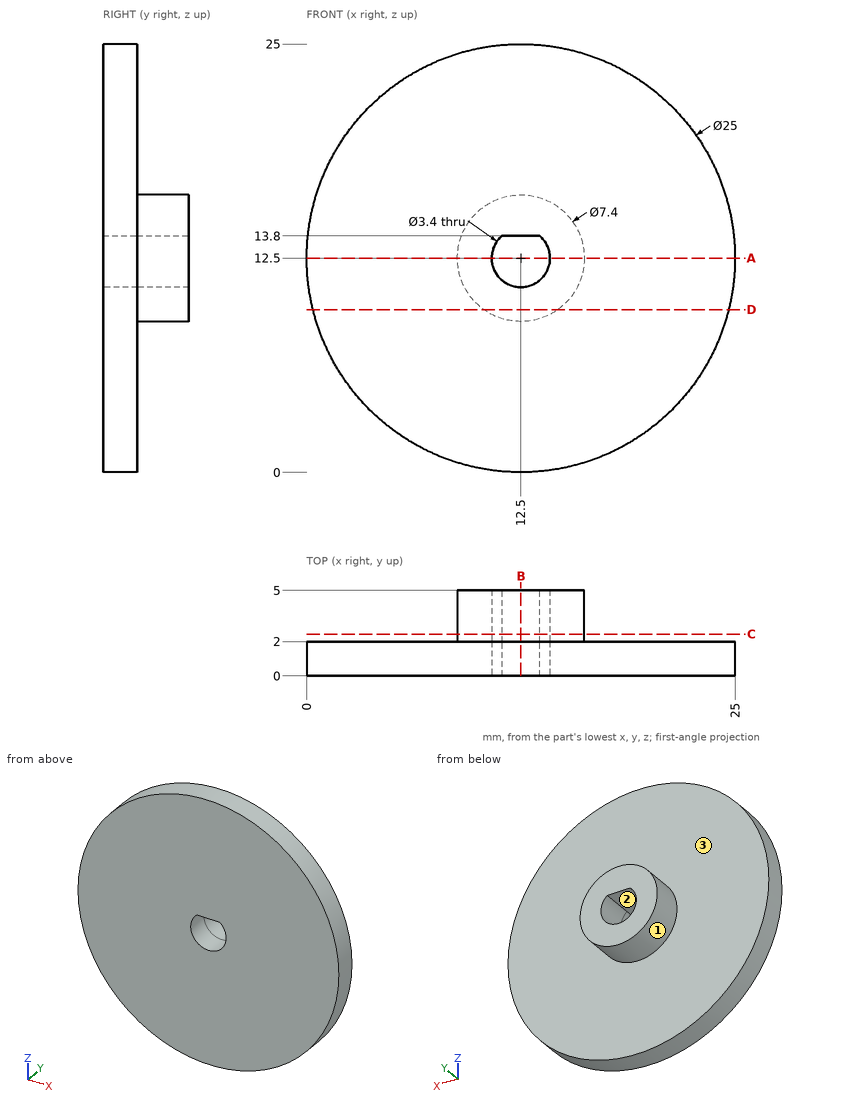
Design review of the part shown in the three views and the two pictorial views. Dimensions are in mm from the part's minimum x, y and z. Round coordinates to 2 decimals unless told otherwise and drop trailing zeros. Loops run counter-clockwise (first coordinate to the right, second up) from the corner with the lowest first, then second, coordinate; pieces in that order, holes last.
Q1. Add section A-A on z = 12.5. Write out the cut boundary in (x, y).
Result sheet:
outline: (0, 0) - (10.8, 0) - (10.8, 5) - (8.8, 5) - (8.8, 2) - (0, 2) - close; (14.2, 0) - (25, 0) - (25, 2) - (16.2, 2) - (16.2, 5) - (14.2, 5) - close
Q2. Add section C-C on y = 2.45. Write out the cut boundary in (x, z), plus the area to 3 significant figures.
Result sheet:
outline: circle Ø7.4 at (12.5, 12.5); hole (11.4, 13.8) arc R1.7 ccw (long way) to (13.6, 13.8) - close
area: 34.5 mm2
Q3. To check wall thickness, follow line 1 along X through (y, z) = (0.8, 12.5); line 2 along X through (y, z) = (3, 12.5); line 3 along Z through (x, y) = (12.5, 3.5). State the ranges of each line that lie inside material, in increasing order.
Result sheet:
line 1: x = 0 to 10.8, 14.2 to 25
line 2: x = 8.8 to 10.8, 14.2 to 16.2
line 3: z = 8.8 to 10.8, 13.8 to 16.2
Q4. Insertion check: pin 1 Ø12.5 at (x, z) = (18, 13.5) entering from +Y; pin 2 Ø1.8 at (x, y) = (13, 3) entering from -Z; pin 3 Ø12 at (x, z) = (5, 5) entering from +Y. Each pin has a flat end and moves straight along its axis. Give the tip position at first contact, or say it passes through.
Result sheet:
pin 1: stops at y = 5
pin 2: stops at z = 8.8
pin 3: stops at y = 2
Q5. Mouldability with a two-part tool opening along X and no side actions: class the marked faces 1, 2 and 3 as +X half, -X half, draft (parallel to the pull), parting line (faces both ways), or undercut.
Result sheet:
face 1: parting line
face 2: undercut
face 3: draft
Q6. Add section B-B on x = 12.5. Write out the cut boundary in (y, z), plus the area to 3 significant figures.
Result sheet:
outline: (0, 0) - (2, 0) - (2, 8.8) - (5, 8.8) - (5, 10.8) - (0, 10.8) - close; (0, 13.8) - (5, 13.8) - (5, 16.2) - (2, 16.2) - (2, 25) - (0, 25) - close
area: 57.2 mm2
Q7. Add section D-D on z = 9.5. Write out the cut boundary in (x, y), plus the area to 3 significant figures.
Result sheet:
outline: (0.37, 0) - (24.63, 0) - (24.63, 2) - (14.67, 2) - (14.67, 5) - (10.33, 5) - (10.33, 2) - (0.37, 2) - close
area: 61.5 mm2
